```python
from build123d import *

# Parameters (mm, degrees)
F2_R     = 0.75
F3_DEPTH = 6
F4_W     = 1
F4_H     = 2
F5_DEPTH = 4


with BuildPart() as f1:
    # F0 (on Front) → F1 (revolve)
    with BuildSketch(Plane.XZ):
        Polygon((2.5, -1.5), (2.5, 0), (8.5725, 0), (8.5725, 23), (3, 23), (3, 24.5), (0, 24.5), (0, -1.5), align=None)
    revolve(axis=Axis((0, 0, 11.5), (0, 0, 1)))

    # F2 (on face) → F3 (join)
    with BuildSketch(Plane.XY.offset(24.5)):
        Circle(F2_R)
    extrude(amount=F3_DEPTH)

    # F4 (on face) → F5 (join)
    with BuildSketch(Plane(origin=(0, 0, 0), x_dir=(1, 0, 0), z_dir=(0, 0, -1))):
        with Locations((5.75, 0)):
            Rectangle(F4_W, F4_H)
        with Locations((-5.75, 0)):
            Rectangle(F4_W, F4_H)
    extrude(amount=F5_DEPTH)


solid = f1.part
```
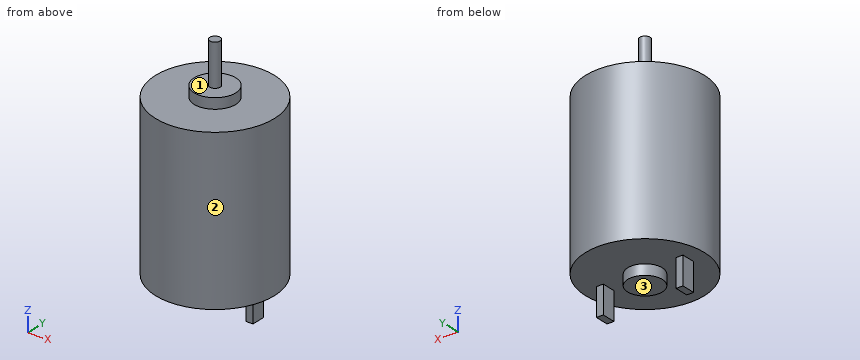
Can you work these out from the model? Positions are in its coordinate system, mm. Face numbers are marked on the shaded views. Coordinates: 2 decimals unless noted, no trailing zeros. Loops run counter-clockwise (first coordinate to the right, second up) from the corner with the lowest first, then second, coordinate; pieces in that order, holes last.
1) Thinking about a two-plate mould opening in Z: for the marked faces 1, 2 and 3, which applies, pulls with the +Z half, pulls with the -Z half, needs draft (parallel to the pull), parting line crosses it, or undercut?
2) Imagine slicing it at C-C on z = 20.5. List the corners of the cut face in (x, y) for me (1 decimal).
3) Imagine slicing it at D-D on x = -1.75. List the corners of the cut face in (y, z) for me.
4) For pin 1 (1.5 mm diameter, centred on x = 0.5, y = -0.5, fed in from -Z); pin 2 (1.1 mm diameter, centred on x = 6, z = -1.5, fed in from -Y); pin 3 (6 mm diameter, centred on x = -5, y = -2.5, fed in from +Z), each with a flat end and sliding along its axis, tell me the tip position at first contact or that it passes through.
5) I need wall thicknesses on probe 1 along Z at (x, y) = (-3, 2.25); probe 2 along Z at (x, y) = (1.5, 2.25); probe 3 along X at (y, z) = (-5.5, 6). Which ranges of each line are inside material? Lowest first, please.
6) Imagine slicing it at B-B on x = 0. List the corners of the cut face in (y, z) for me.
7) Imagine slicing it at A-A on y = 0. List the corners of the cut face in (x, z) for me.
Completed:
1. face 1: pulls with the +Z half
1. face 2: needs draft
1. face 3: pulls with the -Z half
2. outline: circle Ø17.1 at (0, 0)
3. outline: (-8.39, 0) - (-1.79, 0) - (-1.79, -1.5) - (1.79, -1.5) - (1.79, 0) - (8.39, 0) - (8.39, 23) - (2.44, 23) - (2.44, 24.5) - (-2.44, 24.5) - (-2.44, 23) - (-8.39, 23) - close
4. pin 1: stops at z = -1.5
4. pin 2: stops at y = -1
4. pin 3: stops at z = 24.5
5. probe 1: z = 0 to 23
5. probe 2: z = 0 to 24.5
5. probe 3: x = -6.58 to 6.58
6. outline: (-8.57, 0) - (-2.5, 0) - (-2.5, -1.5) - (2.5, -1.5) - (2.5, 0) - (8.57, 0) - (8.57, 23) - (3, 23) - (3, 24.5) - (0.75, 24.5) - (0.75, 30.5) - (-0.75, 30.5) - (-0.75, 24.5) - (-3, 24.5) - (-3, 23) - (-8.57, 23) - close
7. outline: (-8.57, 0) - (-6.25, 0) - (-6.25, -4) - (-5.25, -4) - (-5.25, 0) - (-2.5, 0) - (-2.5, -1.5) - (2.5, -1.5) - (2.5, 0) - (5.25, 0) - (5.25, -4) - (6.25, -4) - (6.25, 0) - (8.57, 0) - (8.57, 23) - (3, 23) - (3, 24.5) - (0.75, 24.5) - (0.75, 30.5) - (-0.75, 30.5) - (-0.75, 24.5) - (-3, 24.5) - (-3, 23) - (-8.57, 23) - close
